```python
from build123d import *

# Parameters (mm, degrees)
F0_R         = 11.2475
F1_DEPTH     = 8
F2_R         = 11
F3_DEPTH     = 7.5
F4_W         = 4.6930826756
F4_H         = 22
F5_DEPTH     = 1.5
F6_T1_DEPTH  = 9.6930826756
F6_T3_DEPTH  = 27
F6_T8_ANGLE  = 90.6971129065
F6_T13_ANGLE = 181.4172742502
F6_T18_ANGLE = 90.6971129065


# Not quite as in the source:
# - a fillet or chamfer that OpenCascade refuses, or shapes differently, is made with other operations: its cross-section is extruded or revolved along the edge and cut away or added


with BuildPart() as f1:
    # F0 (on Front) → F1 (new body)
    with BuildSketch(Plane.XZ):
        Circle(F0_R)
    extrude(amount=F1_DEPTH)

    # F2 (on face) → F3 (cut)
    with BuildSketch(Plane.XZ.offset(8)):
        Circle(F2_R)
    extrude(amount=-F3_DEPTH, mode=Mode.SUBTRACT)

    # F4 (on face) → F5 (join)
    with BuildSketch(Plane(origin=(0, 0, 0), x_dir=(-1, 0, 0), z_dir=(0, 1, 0))):
        Rectangle(F4_W, F4_H)
    extrude(amount=F5_DEPTH)

    # F6: fillet of radius 1 on 9 edges, made by hand

    # F6_s2 → F6_t1 (cut)
    with BuildSketch(Plane.YZ.offset(-4.8465413378)):
        with BuildLine():
            ThreePointArc((0.5, -11), (1.2071067812, -10.7071067812), (1.5, -10))
            Line((1.5, -10), (1.5, -11))
            Line((1.5, -11), (0.5, -11))
        make_face()
        with BuildLine():
            ThreePointArc((0.5, 11), (1.2071067812, 10.7071067812), (1.5, 10))
            Line((1.5, 10), (1.5, 11))
            Line((1.5, 11), (0.5, 11))
        make_face()
    extrude(amount=F6_T1_DEPTH, mode=Mode.SUBTRACT)

    # F6_s4 → F6_t3 (cut)
    with BuildSketch(Plane.XY.offset(-13.5)):
        with BuildLine():
            ThreePointArc((-2.3465413378, 0.5), (-2.053648119, 1.2071067812), (-1.3465413378, 1.5))
            Line((-1.3465413378, 1.5), (-2.3465413378, 1.5))
            Line((-2.3465413378, 1.5), (-2.3465413378, 0.5))
        make_face()
        with BuildLine():
            ThreePointArc((2.3465413378, 0.5), (2.053648119, 1.2071067812), (1.3465413378, 1.5))
            Line((1.3465413378, 1.5), (2.3465413378, 1.5))
            Line((2.3465413378, 1.5), (2.3465413378, 0.5))
        make_face()
    extrude(amount=F6_T3_DEPTH, mode=Mode.SUBTRACT)


with BuildPart() as f6_tool6:
    # F6_s7 → F6_t8 (revolve)
    with BuildSketch(Plane.XY):
        with BuildLine():
            ThreePointArc((11.2475, -1), (10.9546067812, -0.2928932188), (10.2475, 0))
            Line((10.2475, 0), (11.2475, 0))
            Line((11.2475, 0), (11.2475, -1))
        make_face()
    revolve(axis=Axis((0, 0, 0), (0, -1, 0)), revolution_arc=F6_T8_ANGLE)

    split(bisect_by=Plane.YZ.offset(2.3465413378), keep=Keep.TOP)


with BuildPart() as f1_1:
    add(f1.part)

    # F6_t5: cut F6_tool6
    add(f6_tool6.part, mode=Mode.SUBTRACT)


with BuildPart() as f6_tool11:
    # F6_s12 → F6_t13 (revolve)
    with BuildSketch(Plane(origin=(0, 0, 0), x_dir=(0, 1, 0), z_dir=(0.9999235166, 0, -0.0123677357))):
        with BuildLine():
            ThreePointArc((-1, 11.2475), (-0.2928932188, 10.9546067812), (0, 10.2475))
            Line((0, 10.2475), (0, 11.2475))
            Line((0, 11.2475), (-1, 11.2475))
        make_face()
    revolve(axis=Axis((0, 0, 0), (0, -1, 0)), revolution_arc=F6_T13_ANGLE)

    split(bisect_by=Plane.YZ.offset(-2.3465413378), keep=Keep.BOTTOM)


with BuildPart() as f1_2:
    add(f1_1.part)

    # F6_t10: cut F6_tool11
    add(f6_tool11.part, mode=Mode.SUBTRACT)


with BuildPart() as f6_tool16:
    # F6_s17 → F6_t18 (revolve)
    with BuildSketch(Plane(origin=(0, 0, 0), x_dir=(0, 1, 0), z_dir=(-0.999925984, 0, 0.0121666153))):
        with BuildLine():
            ThreePointArc((-1, 11.2475), (-0.2928932188, 10.9546067812), (0, 10.2475))
            Line((0, 10.2475), (0, 11.2475))
            Line((0, 11.2475), (-1, 11.2475))
        make_face()
    revolve(axis=Axis((0, 0, 0), (0, -1, 0)), revolution_arc=F6_T18_ANGLE)

    split(bisect_by=Plane.YZ.offset(2.3465413378), keep=Keep.TOP)


with BuildPart() as f1_3:
    add(f1_2.part)

    # F6_t15: cut F6_tool16
    add(f6_tool16.part, mode=Mode.SUBTRACT)

    # F6_s20 → F6_t21 (revolve, cut)
    with BuildSketch(Plane.XY):
        with BuildLine():
            ThreePointArc((11.2475, -7.3414077513), (11.1835822613, -7.6931889333), (11, -8))
            Line((11, -8), (11.2475, -8))
            Line((11.2475, -8), (11.2475, -7.3414077513))
        make_face()
    revolve(axis=Axis((0, -8, 0), (0, -1, 0)), mode=Mode.SUBTRACT)


solid = f1_3.part
```
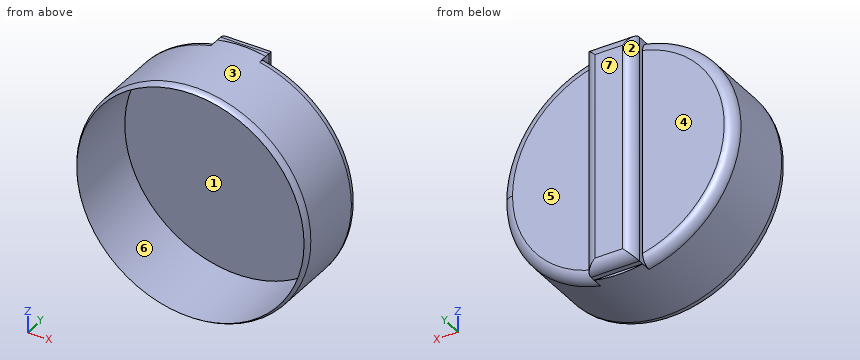
The listing builds one solid part. Answer for the finished solid, in the listing's coordinates (mm). Face numbers are marked on the shaded views. A direction names the side the tool comes from. Round coordinates to 2 decimals unless told otherwise and drop trailing zeros. Write each loop counter-clockwise with the first axis right and the second up, starting at its lowest first coordinate (ties: lowest second). Pieces come first, ordered by that corner, then holes. Notation, with made-up numbers: (-15.5, 21) -> (-4.5, 21) arc R10 ccw to (-4.5, 27) -> close; hole circle Ø1 at (61.25, 36.25). An arc over 180 degrees is marked (long way). Use CSV: the item, a comma, the result in double quotes. Start each with the question number.
(1) The mould has two halves that part along X. Classify the marked faces 1, 2, 3 and 4: released by +X, released by -X, zero draft, split by the parting line, or undercut.
(2) Each of these flat-tipped pins is pushed along its axis until it touches: pin 1 (1.7 mm diameter, centred on y = 0, z = 2.5, fed in from -X); pin 2 (1 mm diameter, centred on x = -4.5, z = -4.5, fed in from -Y); pin 3 (4 mm diameter, centred on x = -3.5, y = -1, fed in from +Z). Where does it stop, or does it pass through?
(3) Section B-B on y = -3.5 is taken. Give the vertices of the cut face in (x, z) (1 decimal), then the cut area to 3 significant figures.
(4) Which of the six approach directions +Z, -Z, +X, -X, +Y, -Y give full straight-line access (tool end or side, diameter ignored) to the marked faces 5, 6 and 7?
(5) Consider L1, parallel to Y at x = 3.25, z = -3.5; L2, parallel to Z at x = 0, y = -6; L3, parallel to X at y = -7.5, z = 5.5. Determine where each line is inside the solid, lowest interval first. Write a range as from..to.
(6) Section A-A on x = 0 is taken. Give the vertices of the cut face in (y, z), then the cut area to 3 significant figures.
A:
1,face 1,"undercut"
1,face 2,"released by -X"
1,face 3,"split by the parting line"
1,face 4,"zero draft"
2,pin 1,"stops at x = -11.02"
2,pin 2,"stops at y = -0.5"
2,pin 3,"stops at z = 11.15"
3,outline,"circle Ø22.5 at (0, 0); hole circle Ø22 at (0, 0)"
3,area,"17.3 mm²"
4,face 5,"+Z, -Z, +X, +Y"
4,face 6,"-Y"
4,face 7,"+Z, -Z, +X, -X, +Y"
5,L1,"y = -0.5..0"
5,L2,"z = -11.25..-11, 11..11.25"
5,L3,"x = -9.8..-9.53, 9.53..9.8"
6,outline,"(-8, -11) arc R1 ccw to (-7.34, -11.25) -> (0, -11.25) -> (0, -11) -> (0.5, -11) arc R1 ccw to (1.5, -10) -> (1.5, 10) arc R1 ccw to (0.5, 11) -> (0, 11) -> (0, 11.25) -> (-7.34, 11.25) arc R1 ccw to (-8, 11) -> (-0.5, 11) -> (-0.5, -11) -> close"
6,area,"47.4 mm²"
